```python
from build123d import *

# Parameters (mm, degrees)
F0_W         = 76.2
F0_H         = 76.2
F1_DEPTH     = 50.8
F2_R         = 12.7
F3_DEPTH     = 76.201
F5_DEPTH     = 25.4
F6_DEPTH     = 50.801
F7_R         = 25.39999
F9_DEPTH     = 25.4
F10_DEPTH    = 76.201
F11_T1_DEPTH = 203.2


# Not quite as in the source:
# - a fillet or chamfer that OpenCascade refuses, or shapes differently, is made with other operations: its cross-section is extruded or revolved along the edge and cut away or added
# - a fillet or chamfer is up to 0.001 mm smaller than in the source, because OpenCascade refuses the exact size


with BuildPart() as f1:
    # F0 (on Front) → F1 (new body)
    with BuildSketch(Plane.XZ):
        with Locations((38.1, 38.1)):
            Rectangle(F0_W, F0_H)
    extrude(amount=F1_DEPTH)

    # F2 (on face) → F3 (cut, through all)
    with BuildSketch(Plane.YZ.offset(76.2)):
        with Locations((-25.4, 25.4)):
            Circle(F2_R)
    extrude(amount=-F3_DEPTH, mode=Mode.SUBTRACT)

    # F4 (on face) → F5 (cut)
    with BuildSketch(Plane.XZ.offset(50.8)):
        Polygon((63.5, 34.925), (76.2, 34.925), (76.2, 76.2), (0, 76.2), (19.05, 50.8), (50.8, 50.8), (50.8, 15.875), (63.5, 15.875), align=None)
    extrude(amount=-F5_DEPTH, mode=Mode.SUBTRACT)

    # F4 (on face) → F6 (cut, through all)
    with BuildSketch(Plane.XZ.offset(50.8)):
        Polygon((63.5, 34.925), (76.2, 34.925), (76.2, 76.2), (0, 76.2), (19.05, 50.8), (50.8, 50.8), (50.8, 15.875), (63.5, 15.875), align=None)
    extrude(amount=-F6_DEPTH, mode=Mode.SUBTRACT)

    # F7 (radius 25.4 in the source; OpenCascade refuses exactly that, so slightly less here)
    f7_edges = [f1.edges().sort_by_distance(p)[0] for p in [
        (34.925, -50.8, 50.8),
        (34.925, 0, 50.8),
    ]]
    fillet(f7_edges, radius=F7_R)

    # F8 (on face) → F9 (cut)
    with BuildSketch(Plane(origin=(0, 0, 0), x_dir=(0, -1, 0), z_dir=(-1, 0, 0))):
        with BuildLine():
            Line((50.8, 76.2), (12.7, 76.2))
            Line((12.7, 76.2), (12.7, 63.5934035911))
            Line((12.7, 63.5934035911), (38.1, 63.5934035911))
            Line((38.1, 63.5934035911), (38.1, 47.3970452561))
            ThreePointArc((38.1, 47.3970452561), (47.3970452561, 38.1), (50.8, 25.4))
            Line((50.8, 25.4), (50.8, 76.2))
        make_face()
    extrude(amount=-F9_DEPTH, mode=Mode.SUBTRACT)

    # F8 (on face) → F10 (cut, through all)
    with BuildSketch(Plane(origin=(0, 0, 0), x_dir=(0, -1, 0), z_dir=(-1, 0, 0))):
        with BuildLine():
            Line((50.8, 76.2), (12.7, 76.2))
            Line((12.7, 76.2), (12.7, 63.5934035911))
            Line((12.7, 63.5934035911), (38.1, 63.5934035911))
            Line((38.1, 63.5934035911), (38.1, 47.3970452561))
            ThreePointArc((38.1, 47.3970452561), (47.3970452561, 38.1), (50.8, 25.4))
            Line((50.8, 25.4), (50.8, 76.2))
        make_face()
    extrude(amount=-F10_DEPTH, mode=Mode.SUBTRACT)

    # F11: fillet of radius 25.4 on 2 edges, made by hand

    # F11_s2 → F11_t1 (cut)
    with BuildSketch(Plane.YZ.offset(-63.5)):
        with BuildLine():
            ThreePointArc((-50.8, 25.4), (-43.3605122421, 7.4394877579), (-25.4, 0))
            Line((-25.4, 0), (-50.8, 0))
            Line((-50.8, 0), (-50.8, 25.4))
        make_face()
        with BuildLine():
            ThreePointArc((0, 25.4), (-7.4394877579, 7.4394877579), (-25.4, 0))
            Line((-25.4, 0), (0, 0))
            Line((0, 0), (0, 25.4))
        make_face()
    extrude(amount=F11_T1_DEPTH, mode=Mode.SUBTRACT)


solid = f1.part
```
Geometry: final body of the model. Coordinates: model frame, mm. A direction names the side the tool comes from. Coordinates: 2 decimals unless noted, no trailing zeros. Loops run counter-clockwise (first coordinate to the right, second up) from the corner with the lowest first, then second, coordinate; pieces in that order, holes last. Notation, with made-up numbers: (38, 66) -> (59, 66) arc R21 ccw to (59, 100) -> close; hole circle Ø10 at (86, -17). An arc over 180 degrees is marked (long way). Use a Markdown table: item, result. Add a question column.
(1) Line query: line 1 along Z through (x, y) = (32, -25.4); line 2 along Y through (x, z) = (16, 25.4); line 3 along Z through (x, y) = (46, -31.5). Output: solid intervals per line, ascending.
(2) Pin query (flat end, axial travel): pin 1 Ø1 at (x, z) = (43.5, 47.5) entering from -Y; pin 2 Ø5 at (x, y) = (30.5, -40) entering from +Z; pin 3 Ø3 at (x, y) = (6.5, -29) entering from +Z. Return the tip coordinate at first contact, or that it passes through.
(3) Mould query, pull axis X, two halves, no side actions, for faces 1 (the flat face through (63.5, -44, 25)), 2 (the cylindrical face through (38.675, -11.061, 46.365)), 3 (the flat face through (70, 0, 30)), 4 (the flat face through (0, -19, 38)). Classes: pulls with the +X half, pulls with the -X half, needs draft (parallel to the pull), parting line crosses it, or undercut.
(4) Access query for faces 5 (the flat face through (63.5, -7, 25)), 6 (the flat face through (70, -9, 34.925)), 7 (the flat face through (8, -38.1, 54)), 8 (the cylindrical face through (35.15, -31.88, 49.96)). Directions: +Z, -Z, +X, -X, +Y, -Y. A direction counts if a zero-diameter tool reaches every point of the face in a straight line with its end or side. Return the directions, or none.
(5) Section query D-D, the plane x = 11. Return loops of the section in (y, z).
(6) Section query A-A, the plane y = -14.5. Return loops of the section in (x, z) (3 decimals), plus the area to 3 significant figures.
(7) Section query B-B, the plane z = 32. Return loops of the section in (x, y), plus the area to 3 significant figures.
(8) Section query C-C, the plane y = -31. Return loops of the section in (x, z).
Answer:
| question | item | result |
|---|---|---|
| 1 | line 1 | z = 0 to 12.7, 38.1 to 50.8 |
| 1 | line 2 | y = -50.8 to -38.1, -12.7 to 0 |
| 1 | line 3 | z = 0.74 to 14.26, 36.54 to 50.06 |
| 2 | pin 1 | stops at y = -38.76 |
| 2 | pin 2 | stops at z = 47.73 |
| 2 | pin 3 | stops at z = 63.59 |
| 3 | face 1 | undercut |
| 3 | face 2 | undercut |
| 3 | face 3 | needs draft |
| 3 | face 4 | pulls with the -X half |
| 4 | face 5 | +Z, +Y, -Y |
| 4 | face 6 | +Z, +X, +Y, -Y |
| 4 | face 7 | +Z, +X, -X, -Y |
| 4 | face 8 | +Z, +X, -Y |
| 5 | outline | (-38.1, 47.4) arc R25.4 ccw (long way) to (0, 25.4) -> (0, 61.53) -> (-38.1, 61.53) -> close; hole circle Ø25.4 at (-25.4, 25.4) |
| 6 | outline | (0, 2.458) -> (76.2, 2.458) -> (76.2, 18.882) -> (63.5, 18.882) -> (63.5, 15.875) -> (50.8, 15.875) -> (50.8, 18.882) -> (0, 18.882) -> close; (0, 31.918) -> (50.8, 31.918) -> (50.8, 48.342) -> (20.893, 48.342) -> (9.455, 63.593) -> (0, 63.593) -> close; (63.5, 31.918) -> (76.2, 31.918) -> (76.2, 34.925) -> (63.5, 34.925) -> close |
| 6 | area | 2,320 mm^2 |
| 7 | outline | (0, -49.93) -> (50.8, -49.93) -> (50.8, -36.25) -> (0, -36.25) -> close; (0, -14.55) -> (50.8, -14.55) -> (50.8, -0.87) -> (33.15, -0.87) -> (33.15, 0) -> (0, 0) -> close; (63.5, -49.93) -> (76.2, -49.93) -> (76.2, -36.25) -> (63.5, -36.25) -> close; (63.5, -14.55) -> (76.2, -14.55) -> (76.2, 0) -> (63.5, 0) -> close |
| 7 | area | 1,780 mm^2 |
| 8 | outline | (0, 0.63) -> (76.2, 0.63) -> (76.2, 14) -> (0, 14) -> close; (0, 36.8) -> (50.8, 36.8) -> (50.8, 50.17) -> (19.52, 50.17) -> (9.45, 63.59) -> (0, 63.59) -> close |
